Part model, mm, in its own coordinate system. Round coordinates to 2 decimals unless told otherwise and drop trailing zeros. Order: outer loops, then holes, each group sorted by start corner. A loop starts at its lowest first (then second) coordinate and runs counter-clockwise, first axis right, second up. Notation, with made-up numbers: (28, 61) -> (68, 61) arc R7 cw to (68, 74) -> close; hole circle Ø6 at (44, 0.25). An arc over 180 degrees is marked (long way). Return JSON: item names as keys, results as strings. Group by question number.
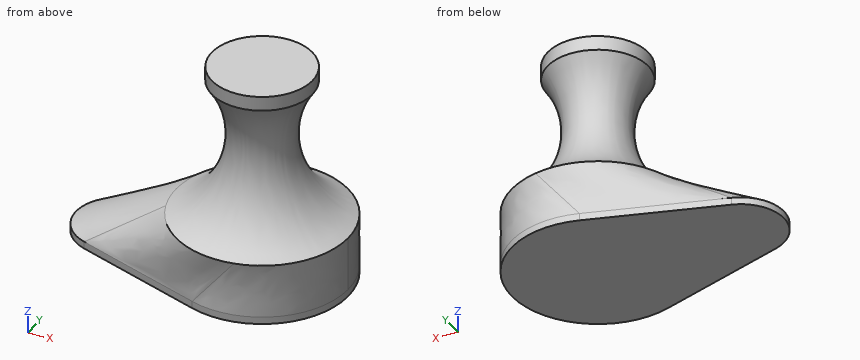
from build123d import *

# Parameters (mm, degrees)
SKETCH002_R  = 12
PAD_DEPTH    = 1
SKETCH001_R  = 7.75
POCKET_DEPTH = 5.75


with BuildPart() as part:
    # Sketch → Revolution (revolve)
    with BuildSketch(Plane.XZ):
        with BuildLine():
            ThreePointArc((7, 27.944074), (4.909607, 17.041628), (12, 8.5))
            Line((12, 8.5), (0, 8.5))
            Line((0, 8.5), (0, 29.944074))
            Line((7, 29.944074), (0, 29.944074))
            Line((7, 27.944074), (7, 29.944074))
        make_face()
    revolve(axis=Axis((0, 0, 0), (0, 0, 1)))

    # Sketch002 (on DatumPlane) → AdditiveLoft section 0
    with BuildSketch(Plane(origin=(0, 0, 8.5), x_dir=(1, 0, 0), z_dir=(0, 0, -1))):
        Circle(SKETCH002_R)
    # Sketch004 → AdditiveLoft section 1
    with BuildSketch(Plane.XY.offset(1)):
        with BuildLine():
            ThreePointArc((-3.6, -11.44727), (12, 0), (-3.6, 11.44727))
            Line((-21.8, 5.723635), (-3.6, 11.44727))
            ThreePointArc((-21.8, 5.723635), (-26, 0), (-21.8, -5.723635))
            Line((-21.8, -5.723635), (-3.6, -11.44727))
        make_face()
    loft(ruled=True)

    # Sketch003 → Pad (new body)
    with BuildSketch(Plane.XY):
        with BuildLine():
            ThreePointArc((-3.6, -11.44727), (12, 0), (-3.6, 11.44727))
            Line((-21.8, 5.723635), (-3.6, 11.44727))
            ThreePointArc((-21.8, 5.723635), (-26, 0), (-21.8, -5.723635))
            Line((-21.8, -5.723635), (-3.6, -11.44727))
        make_face()
    extrude(amount=PAD_DEPTH)

    # Sketch001 → Pocket (cut)
    with BuildSketch(Plane.XY.offset(0.5)):
        Circle(SKETCH001_R)
    extrude(amount=POCKET_DEPTH, mode=Mode.SUBTRACT)


solid = part.part
(1) Pin check, flat tips, straight feed: P1, Ø5, axis at x = -19.5, z = 7.5, coming from the -Y side; P2, Ø4, axis at y = 1.5, z = 26, coming from the -X side; P3, Ø2, axis at y = -8, z = 6, coming from the -X side; P4, Ø8, axis at x = -3.5, z = 20, coming from the -Y side. Stop position of each tip, or through.
(2) Saw through at C-C, the plane z = 10.25. List the corners of the cut face in (x, y).
(3) Probe L1, parallel to Z at x = -1, y = -3.5; L2, parallel to Z at x = 1.5, y = -6; L3, parallel to Z at x = 5, y = -4.75. List the from-to ranges inside material, lowest first. Write a range as [from, to].
(4) Saw through at B-B, the plane z = 19.75. List the corners of the cut face in (x, y), and give its area (3 significant figures).
(5) Saw through at A-A, the plane y = -6.5. State how many separate pieces and enclosed holes the cut face has, and give its area (3 significant figures).
Results are:
{
 "1": {"P1": "passes through", "P2": "stops at x = -6.92", "P3": "stops at x = -12.92", "P4": "stops at y = -4.85"},
 "2": {"outline": "circle Ø18.46 at (0, 0)"},
 "3": {"L1": "z = [0, 0.5], [6.25, 29.94]", "L2": "z = [0, 0.5], [6.25, 13.88], [26.68, 29.94]", "L3": "z = [0, 0.5], [6.25, 12.76], [27.8, 29.94]"},
 "4": {"outline": "circle Ø9.02 at (0, 0)", "area": "63.9 mm^2"},
 "5": {"separate pieces": "2", "enclosed holes": "1", "area": "232 mm^2"}
}
